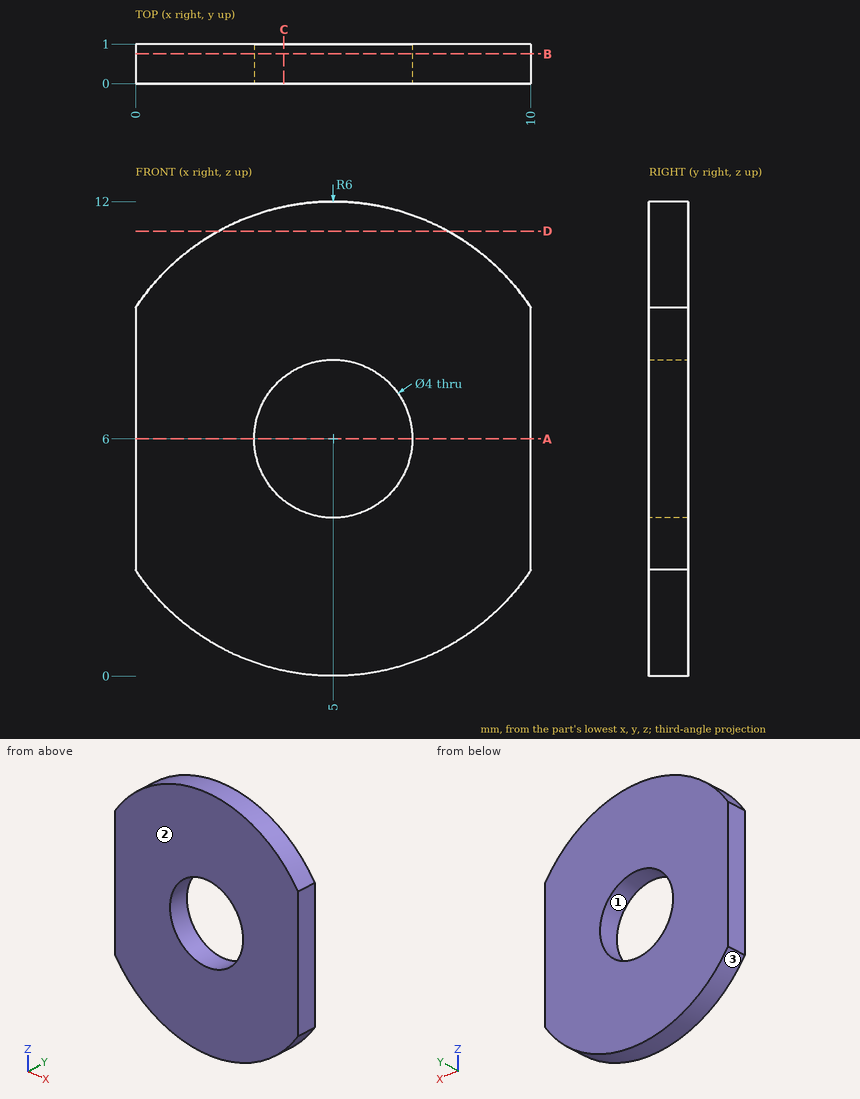
Verification items for this drawing (mm, ordinates from the low corner). Coordinates: 2 decimals unless noted, no trailing zeros. Write each loop counter-clockwise with the first axis right and the second up, starting at its lowest first coordinate (ties: lowest second). Pieces come first, ordered by that corner, then holes. Notation, with made-up numbers: M 4.25,-11 L 40.25,-11 A24 ccw 40.25,28 Z; hole C 57,9.5 d5. An arc over 180 degrees is marked long. Answer as a JSON object with one key per item and string values. Group by question number.
(1) Cross-section at D-D, the plane z = 11.25. Record the cut outline in (x, y), and give its area (3 significant figures).
(2) Release check for a two-part mould opening along X. For the marked faces 1, 2 and 3 record: +X half, -X half, draft (parallel to the pull), parting line (faces both ways), or undercut.
(3) Cross-section at A-A, the plane z = 6. Record the cut outline in (x, y), and give its area (3 significant figures).
(4) Cross-section at B-B, the plane y = 0.75. Record the cut outline in (x, z).
(5) Material ranges on line 1 (X direction, y = 0.4, z = 6); line 2 (X direction, y = 0.9, z = 4.75); line 3 (Z direction, x = 7.25, y = 0.7), recorded low to high.
(6) Cross-section at C-C, the plane x = 3.75. Record the cut outline in (y, z), and give its area (3 significant figures).
Reply:
{
 "1": {"outline": "M 2.1,0 L 7.9,0 L 7.9,1 L 2.1,1 Z", "area": "5.81 mm²"},
 "2": {"face 1": "undercut", "face 2": "draft", "face 3": "parting line"},
 "3": {"outline": "M 0,0 L 3,0 L 3,1 L 0,1 Z; M 7,0 L 10,0 L 10,1 L 7,1 Z", "area": "6.00 mm²"},
 "4": {"outline": "M 0,2.68 A6 ccw 10,2.68 L 10,9.32 A6 ccw 0,9.32 Z; hole C 5,6 d4"},
 "5": {"line 1": "0 to 3, 7 to 10", "line 2": "0 to 3.44, 6.56 to 10", "line 3": "0.44 to 11.56"},
 "6": {"outline": "M 0,0.13 L 1,0.13 L 1,4.44 L 0,4.44 Z; M 0,7.56 L 1,7.56 L 1,11.87 L 0,11.87 Z", "area": "8.61 mm²"}
}
